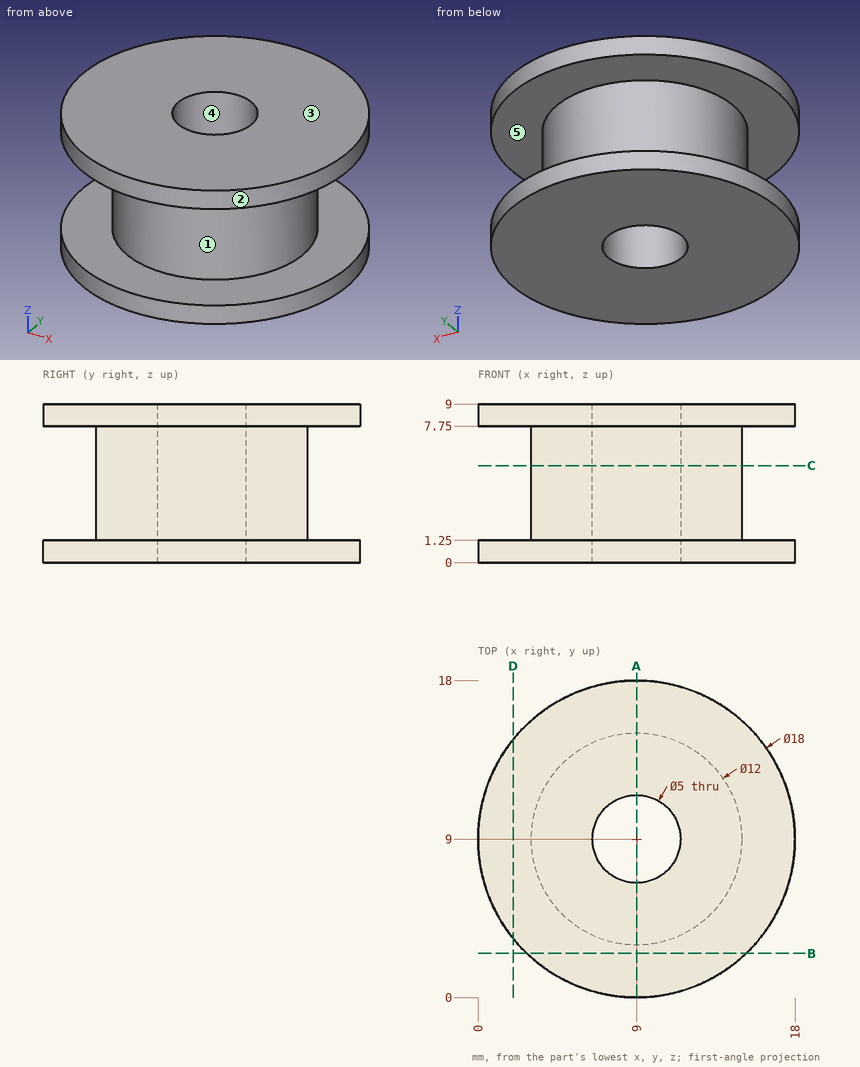
Print and shaded views of the part. All mm, measured from the part's lowest x, y and z. A direction names the side the tool comes from. Round coordinates to 2 decimals unless told otherwise and drop trailing zeros. Write each loop counter-clockwise with the first axis right and the second up, starting at its lowest first coordinate (ties: lowest second). Pieces come first, ordered by that corner, then holes. Notation, with made-up numbers: (45, 75) - (68, 75) arc R17 cw to (68, 93) - close; hole circle Ø1 at (28, 28.5). An arc over 180 degrees is marked (long way). Use CSV: the item, a comma, the result in double quotes. Start each with the question number.
Item 1: Drill centre lines: L1, parallel to Z at x = 5.75, y = 14.5; L2, parallel to Y at x = 9, z = 2.75; L3, parallel to X at y = 10, z = 0.75. Where is each one in solid material? Low to high. Write a range as [from, to].
Item 2: Band-saw the part on A-A (x = 9). Write the cut outline in (y, z).
Item 3: Band-saw the part on C-C (z = 5.5). Write the cut outline in (x, y), and give its area (3 significant figures).
Item 4: Two-plate mould, pull along Z, no slides. Class the marked faces 1, 2 and 3: released by +Z, released by -Z, zero draft, split by the parting line, or undercut.
Item 5: Pin check, flat tips, straight feed: P1, Ø3, axis at y = 3, z = 1, coming from the +X side; P2, Ø4, axis at x = 3, z = 8, coming from the +Y side; P3, Ø8, axis at x = 9, y = 9, coming from the -Z side; P4, Ø4, axis at y = 6.5, z = 6.5, coming from the +X side. Stop position of each tip, or through.
Item 6: Band-saw the part on B-B (y = 2.5). Write the cut outline in (x, z).
Item 7: Band-saw the part on D-D (x = 2). Write the cut outline in (y, z), and give its area (3 significant figures).
Item 8: Tool access for the marked faces 4 and 5: list every direction of +Z, -Z, +X, -X, +Y, -Y with a clear straight run to the whole face (end or side of a thin tool).
Checked values:
1,L1,"z = [0, 1.25], [7.75, 9]"
1,L2,"y = [3, 6.5], [11.5, 15]"
1,L3,"x = [0.06, 6.71], [11.29, 17.94]"
2,outline,"(0, 0) - (6.5, 0) - (6.5, 9) - (0, 9) - (0, 7.75) - (3, 7.75) - (3, 1.25) - (0, 1.25) - close; (11.5, 0) - (18, 0) - (18, 1.25) - (15, 1.25) - (15, 7.75) - (18, 7.75) - (18, 9) - (11.5, 9) - close"
3,outline,"circle Ø12 at (9, 9); hole circle Ø5 at (9, 9)"
3,area,"93.5 mm²"
4,face 1,"undercut"
4,face 2,"zero draft"
4,face 3,"released by +Z"
5,P1,"stops at x = 16.79"
5,P2,"stops at y = 17.06"
5,P3,"stops at z = 0"
5,P4,"stops at x = 17.95"
6,outline,"(2.78, 0) - (15.22, 0) - (15.22, 1.25) - (2.78, 1.25) - close; (2.78, 7.75) - (15.22, 7.75) - (15.22, 9) - (2.78, 9) - close"
7,outline,"(3.34, 0) - (14.66, 0) - (14.66, 1.25) - (3.34, 1.25) - close; (3.34, 7.75) - (14.66, 7.75) - (14.66, 9) - (3.34, 9) - close"
7,area,"28.3 mm²"
8,face 4,"+Z, -Z"
8,face 5,"none"
